from build123d import *

# Parameters (mm, degrees)
SKETCH1_W           = 300
SKETCH1_H           = 400
BOSS_EXTRUDE1_DEPTH = 6
SKETCH2_W           = 6
SKETCH2_H           = 400
BOSS_EXTRUDE2_DEPTH = 300
SKETCH3_W           = 200
SKETCH3_H           = 6
BOSS_EXTRUDE3_DEPTH = 450
SKETCH5_W           = 200
SKETCH5_H           = 150
BOSS_EXTRUDE4_DEPTH = 6


with BuildPart() as part:
    # Sketch1 → Boss-Extrude1 (new body)
    with BuildSketch(Plane(origin=(0, 0, 0), x_dir=(1, 0, 0), z_dir=(0, 1, 0))):
        Rectangle(SKETCH1_W, SKETCH1_H)
    extrude(amount=BOSS_EXTRUDE1_DEPTH)

    # Sketch2 → Boss-Extrude2 (add)
    with BuildSketch(Plane(origin=(0, 6, 0), x_dir=(1, 0, 0), z_dir=(0, 1, 0))):
        with Locations((-137, 0)):
            Rectangle(SKETCH2_W, SKETCH2_H)
    extrude(amount=BOSS_EXTRUDE2_DEPTH)

    # Sketch3 → Boss-Extrude3 (add)
    with BuildSketch(Plane(origin=(0, 6, 0), x_dir=(1, 0, 0), z_dir=(0, 1, 0))):
        with Locations((-34, 187)):
            Rectangle(SKETCH3_W, SKETCH3_H)
    extrude(amount=BOSS_EXTRUDE3_DEPTH)

    # Sketch5 → Boss-Extrude4 (add)
    with BuildSketch(Plane(origin=(0, 456, 0), x_dir=(1, 0, 0), z_dir=(0, 1, 0))):
        with Locations((-34, 125)):
            Rectangle(SKETCH5_W, SKETCH5_H)
    extrude(amount=BOSS_EXTRUDE4_DEPTH)


solid = part.part
Could you check a few things on this model? Use its own coordinates, in mm. A direction names the side the tool comes from. Give positions to 0.01 mm unless a question says otherwise; leave off trailing zeros. Order: outer loops, then holes, each group sorted by start corner. A loop starts at its lowest first (then second) coordinate and runs counter-clockwise, first axis right, second up. Notation, with made-up numbers: (-15.5, -13) -> (29.5, -13) arc R16 cw to (29.5, -2) -> close; hole circle Ø4 at (-18.75, 30.25). An arc over 180 degrees is marked (long way). Answer in a Markdown table with one row per item. Add a question column.
Item 1: Imagine slicing it at D-D (z = 168). List the corners of the cut face in (x, y) for me, and give its area (3 significant figures).
Item 2: We'd pull the mould along Y, two halves only. Please class faces 6 (the flat face through (-35, 228, -190)), 7 (the flat face through (6, 6, -3)), 8 (the flat face through (-2, 0, -3)), 9 (the flat face through (-140, 154, 3)): pulls with the +Y half, pulls with the -Y half, needs draft (parallel to the pull), parting line crosses it, or undercut.
Item 3: I'm going to push flat-ended pins straight in: P1, Ø3, axis at x = -136, z = -19, coming from the +Y side; P2, Ø5, axis at x = -143, z = -59, coming from the +Y side; P3, Ø5, axis at y = 223, z = 160, coming from the -X side. Where does each tip first touch, or does it pass through?
Item 4: Please list where these lines run through material, in increasing order: probe 1 along Y at (x, z) = (22.5, -69); probe 2 along X at (y, z) = (160, -81.5); probe 3 along Y at (x, z) = (79.5, -122.5).
Item 5: For faces 1 (the flat face through (-35, 456, -118)), 2 (the flat face through (-35, 462, -126)), 3 (the flat face through (-134, 418, -186)), 4 (the flat face through (-134, 154, 11)), 5 (the flat face through (66, 233, -186)), which set-ups out of +Z, -Z, +X, -X, +Y, -Y let a thin tool reach every point of the face, with its end or its side?
Item 6: Imagine slicing it at C-C (y = 285). List the corners of the cut face in (x, z) for me, and give its area (3 significant figures).
Item 7: Imagine slicing it at B-B (x = -24). List the corners of the cut face in (y, z) for me.
Item 8: Imagine slicing it at A-A (z = -82). List the corners of the cut face in (x, y) for me.
Result:
| question | item | result |
|---|---|---|
| 1 | outline | (-150, 0) -> (150, 0) -> (150, 6) -> (-134, 6) -> (-134, 306) -> (-140, 306) -> (-140, 6) -> (-150, 6) -> close |
| 1 | area | 3,600 mm2 |
| 2 | face 6 | undercut |
| 2 | face 7 | undercut |
| 2 | face 8 | pulls with the -Y half |
| 2 | face 9 | needs draft |
| 3 | P1 | y = 306 |
| 3 | P2 | y = 6 |
| 3 | P3 | x = -140 |
| 4 | probe 1 | 0 to 6, 456 to 462 |
| 4 | probe 2 | -140 to -134 |
| 4 | probe 3 | 0 to 6 |
| 5 | face 1 | +Z, +X, -X |
| 5 | face 2 | +Z, -Z, +X, -X, +Y |
| 5 | face 3 | +Z, -Z, -X, +Y |
| 5 | face 4 | +Z, +X |
| 5 | face 5 | +Z, -Z, +X, +Y |
| 6 | outline | (-140, -200) -> (-134, -200) -> (-134, -190) -> (66, -190) -> (66, -184) -> (-134, -184) -> (-134, 200) -> (-140, 200) -> close |
| 6 | area | 3,600 mm2 |
| 7 | outline | (0, -200) -> (6, -200) -> (6, -190) -> (456, -190) -> (456, -200) -> (462, -200) -> (462, -50) -> (456, -50) -> (456, -184) -> (6, -184) -> (6, 200) -> (0, 200) -> close |
| 8 | outline | (-150, 0) -> (150, 0) -> (150, 6) -> (-134, 6) -> (-134, 306) -> (-140, 306) -> (-140, 6) -> (-150, 6) -> close; (-134, 456) -> (66, 456) -> (66, 462) -> (-134, 462) -> close |
